```python
from build123d import *

# Parameters (mm, degrees)
SKETCH1_W           = 100
SKETCH1_H           = 40.64
BOSS_EXTRUDE1_DEPTH = 7.5
SKETCH2_W           = 100
SKETCH2_H           = 7.5
BOSS_EXTRUDE2_DEPTH = 46.92
BOSS_EXTRUDE3_DEPTH = 100
FILLET1_R           = 10
FILLET2_R           = 15
FILLET3_R           = 22.5


with BuildPart() as part:
    # Sketch1 → Boss-Extrude1 (new body)
    with BuildSketch(Plane(origin=(0, 0, 0), x_dir=(1, 0, 0), z_dir=(0, 1, 0))):
        Rectangle(SKETCH1_W, SKETCH1_H)
    extrude(amount=BOSS_EXTRUDE1_DEPTH)

    # Sketch2 → Boss-Extrude2 (add)
    with BuildSketch(Plane(origin=(0, 7.5, 0), x_dir=(1, 0, 0), z_dir=(0, 1, 0))):
        with Locations((0, -24.07)):
            Rectangle(SKETCH2_W, SKETCH2_H)
    extrude(amount=-BOSS_EXTRUDE2_DEPTH)

    # Sketch3 → Boss-Extrude3 (add)
    with BuildSketch(Plane.ZY.offset(50)):
        Polygon((20.32, -39.42), (20.32, -42.16), (27.82, -39.42), (27.82, -32.266971567), (20.32, -32.266971567), align=None)
    extrude(amount=-BOSS_EXTRUDE3_DEPTH)

    # Fillet1
    # the kernel refuses this fillet: 10 mm, written as the material it takes off along each edge
    with BuildSketch(Plane(origin=(-74.206145914, 7.5, -20.32), x_dir=(0, -1, 0), z_dir=(1, 0, 0))) as fillet1_piece_1:
        with BuildLine():
            CenterArc((10, -9.682458366), FILLET1_R, 104.477512186, 75.522487814)
            Line((0, -9.682458366), (-0.2, -9.682458366))
            Line((-0.2, -9.682458366), (-0.2, 0))
            Line((-0.2, 0), (0, 0.2))
            ThreePointArc((0, 0.2), (3.75, 0.2), (7.45, 0.193649167))
            Line((7.45, 0.193649167), (7.5, 0))
        make_face()
    extrude(amount=148.412291828, mode=Mode.SUBTRACT)

    # Fillet2
    fillet2_edges = [part.edges().sort_by_distance(p)[0] for p in [
        (0, 0, 20.32),
    ]]
    fillet(fillet2_edges, radius=FILLET2_R)

    # Fillet3
    fillet3_edges = [part.edges().sort_by_distance(p)[0] for p in [
        (0, 7.5, 27.82),
    ]]
    fillet(fillet3_edges, radius=FILLET3_R)


solid = part.part
```
CAD build for the part. Positions are in the model's coordinates, mm. A direction names the side the tool comes from. Give positions to 0.01 mm unless a question says otherwise; leave off trailing zeros. Write each loop counter-clockwise with the first axis right and the second up, starting at its lowest first coordinate (ties: lowest second). Pieces come first, ordered by that corner, then holes. Notation, with made-up numbers: M 86.25,-36.75 L 109.25,-36.75 A32 ccw 109.25,-10.75 Z; hole C -2.75,-25.75 d5. An arc over 180 degrees is marked long. Return JSON: item names as keys, results as strings. Group by question number.
(1) Drill centre lines: L1, parallel to Z at x = 5, y = -20.5; L2, parallel to Y at x = -17, z = -6.5; L3, parallel to Y at x = 29.5, z = 14. Where is each one in solid material? Low to high. Write a range as [from, to].
(2) Flat gauge pins, fed straight in: pin 1 Ø6 at (x, z) = (-11, 19) entering from +Y; pin 2 Ø1 at (x, z) = (8.5, 17) entering from +Y; pin 3 Ø1.5 at (x, y) = (-4.5, -27) entering from -Z. Where does each tip first touch, or does it go through?
(3) 3-axis set-ups, long thin cutter, end or side, ignore diameter. For faces 1 (the face through (-1, -27, 27.82)), 2 (the face through (-1, -28, 20.32)): which of +Z, -Z, +X, -X, +Y, -Y reach the whole face in a straight line?
(4) Band-saw the part on C-C (z = -8). Give the cut face in (x, y).
(5) Band-saw the part on B-B (y = -22). Give the cut face in (x, z).
(6) Band-saw the part on A-A (x = -17.5). Give the cut face in (y, z).
Entries:
{
 "1": {"L1": "z = [20.32, 27.82]", "L2": "y = [0, 7.5]", "L3": "y = [-2.77, 5.76]"},
 "2": {"pin 1": "stops at y = 4.8", "pin 2": "stops at y = 4.53", "pin 3": "stops at z = 20.32"},
 "3": {"face 1": "+Z, +X, -X, +Y, -Y", "face 2": "-Z, +X, -X, -Y"},
 "4": {"outline": "M -50,0 L 50,0 L 50,7.5 L -50,7.5 Z"},
 "5": {"outline": "M -50,20.32 L 50,20.32 L 50,27.82 L -50,27.82 Z"},
 "6": {"outline": "M -42.16,20.32 L -15,20.32 A15 cw 0,5.32 L 0,-20.32 A10 ccw 7.5,-10.64 L 7.5,5.32 A22.5 ccw -15,27.82 L -39.42,27.82 Z"}
}
